from build123d import *

# Parameters (mm, degrees)
BOSS_EXTRUDE3_DEPTH = 3
SKETCH1_5_R         = 8
BOSS_EXTRUDE4_DEPTH = 6
SKETCH1_6_R         = 8
BOSS_EXTRUDE5_DEPTH = 18
SKETCH1_7_R         = 6
CUT_EXTRUDE1_DEPTH  = 12
SKETCH1_8_R         = 3
CUT_EXTRUDE2_DEPTH  = 125


with BuildPart() as part:
    # Sketch1 → Boss-Extrude3 (new body)
    with BuildSketch(Plane(origin=(0, 0, 0), x_dir=(1, 0, 0), z_dir=(0, 1, 0))):
        with BuildLine():
            ThreePointArc((42.894958583, -3.003752345), (37.239092363, 21.5), (18.846153454, 38.65))
            ThreePointArc((18.846153454, 38.65), (16.147655157, 40.973517523), (14.941453584, 44.323995772))
            ThreePointArc((14.941453584, 44.323995772), (0, 58), (-14.941453584, 44.323995772))
            ThreePointArc((-14.941453584, 44.323995772), (-16.147655157, 40.973517523), (-18.846153454, 38.65))
            ThreePointArc((-18.846153454, 38.65), (-37.239092363, 21.5), (-42.894958583, -3.003752345))
            ThreePointArc((-42.894958583, -3.003752345), (-43.557934635, -6.502479184), (-45.856433127, -9.222319513))
            ThreePointArc((-45.856433127, -9.222319513), (-50.229473419, -29), (-30.914979544, -35.101676259))
            ThreePointArc((-30.914979544, -35.101676259), (-27.410279478, -34.471038339), (-24.048805129, -35.646247655))
            ThreePointArc((-24.048805129, -35.646247655), (0, -43), (24.048805129, -35.646247655))
            ThreePointArc((24.048805129, -35.646247655), (27.410279478, -34.471038339), (30.914979544, -35.101676259))
            ThreePointArc((30.914979544, -35.101676259), (50.229473419, -29), (45.856433127, -9.222319513))
            ThreePointArc((45.856433127, -9.222319513), (43.557934635, -6.502479184), (42.894958583, -3.003752345))
        make_face()
        with BuildLine():
            ThreePointArc((-17.531305538, 35.953488372), (-34.641016151, 20), (-39.902287054, -2.794188228))
            ThreePointArc((-39.902287054, -2.794188228), (-40.8493957, -7.792369426), (-44.132964974, -11.67785561))
            ThreePointArc((-44.132964974, -11.67785561), (-47.631397208, -27.5), (-32.179802107, -32.381341007))
            ThreePointArc((-32.179802107, -32.381341007), (-27.173087728, -31.480429693), (-22.370981516, -33.159300144))
            ThreePointArc((-22.370981516, -33.159300144), (0, -40), (22.370981516, -33.159300144))
            ThreePointArc((22.370981516, -33.159300144), (27.173087728, -31.480429693), (32.179802107, -32.381341007))
            ThreePointArc((32.179802107, -32.381341007), (47.631397208, -27.5), (44.132964974, -11.67785561))
            ThreePointArc((44.132964974, -11.67785561), (40.8493957, -7.792369426), (39.902287054, -2.794188228))
            ThreePointArc((39.902287054, -2.794188228), (34.641016151, 20), (17.531305538, 35.953488372))
            ThreePointArc((17.531305538, 35.953488372), (13.676307972, 39.272799119), (11.953162867, 44.059196617))
            ThreePointArc((11.953162867, 44.059196617), (0, 55), (-11.953162867, 44.059196617))
            ThreePointArc((-11.953162867, 44.059196617), (-13.676307972, 39.272799119), (-17.531305538, 35.953488372))
        make_face(mode=Mode.SUBTRACT)
    extrude(amount=BOSS_EXTRUDE3_DEPTH)

    # Sketch1<5> → Boss-Extrude4 (add)
    with BuildSketch(Plane(origin=(0, 0, 0), x_dir=(1, 0, 0), z_dir=(0, 1, 0))):
        with BuildLine():
            ThreePointArc((-17.531305538, 35.953488372), (-13.676307972, 39.272799119), (-11.953162867, 44.059196617))
            ThreePointArc((-11.953162867, 44.059196617), (0, 55), (11.953162867, 44.059196617))
            ThreePointArc((11.953162867, 44.059196617), (13.676307972, 39.272799119), (17.531305538, 35.953488372))
            ThreePointArc((17.531305538, 35.953488372), (34.641016151, 20), (39.902287054, -2.794188228))
            ThreePointArc((39.902287054, -2.794188228), (40.8493957, -7.792369426), (44.132964974, -11.67785561))
            ThreePointArc((44.132964974, -11.67785561), (47.631397208, -27.5), (32.179802107, -32.381341007))
            ThreePointArc((32.179802107, -32.381341007), (27.173087728, -31.480429693), (22.370981516, -33.159300144))
            ThreePointArc((22.370981516, -33.159300144), (0, -40), (-22.370981516, -33.159300144))
            ThreePointArc((-22.370981516, -33.159300144), (-27.173087728, -31.480429693), (-32.179802107, -32.381341007))
            ThreePointArc((-32.179802107, -32.381341007), (-47.631397208, -27.5), (-44.132964974, -11.67785561))
            ThreePointArc((-44.132964974, -11.67785561), (-40.8493957, -7.792369426), (-39.902287054, -2.794188228))
            ThreePointArc((-39.902287054, -2.794188228), (-34.641016151, 20), (-17.531305538, 35.953488372))
        make_face()
        with Locations((37.239092363, -21.5)):
            Circle(SKETCH1_5_R, mode=Mode.SUBTRACT)
        with Locations((-37.239092363, -21.5)):
            Circle(SKETCH1_5_R, mode=Mode.SUBTRACT)
        with Locations((0, 43)):
            Circle(SKETCH1_5_R, mode=Mode.SUBTRACT)
    extrude(amount=BOSS_EXTRUDE4_DEPTH)

    # Sketch1<6> → Boss-Extrude5 (add)
    with BuildSketch(Plane(origin=(0, 0, 0), x_dir=(1, 0, 0), z_dir=(0, 1, 0))):
        with Locations((0, 43)):
            Circle(SKETCH1_6_R)
        with Locations((-37.239092363, -21.5)):
            Circle(SKETCH1_6_R)
        with Locations((37.239092363, -21.5)):
            Circle(SKETCH1_6_R)
    extrude(amount=BOSS_EXTRUDE5_DEPTH)

    # Sketch1<7> → Cut-Extrude1 (cut)
    with BuildSketch(Plane(origin=(0, 0, 0), x_dir=(1, 0, 0), z_dir=(0, 1, 0))):
        with Locations((0, 43)):
            Circle(SKETCH1_7_R)
        with Locations((37.239092363, -21.5)):
            Circle(SKETCH1_7_R)
        with Locations((-37.239092363, -21.5)):
            Circle(SKETCH1_7_R)
    extrude(amount=CUT_EXTRUDE1_DEPTH, mode=Mode.SUBTRACT)

    # Sketch1<8> → Cut-Extrude2 (cut)
    with BuildSketch(Plane(origin=(0, 0, 0), x_dir=(1, 0, 0), z_dir=(0, 1, 0))):
        with Locations((0, 43)):
            Circle(SKETCH1_8_R)
        with Locations((-37.239092363, -21.5)):
            Circle(SKETCH1_8_R)
        with Locations((37.239092363, -21.5)):
            Circle(SKETCH1_8_R)
    extrude(amount=CUT_EXTRUDE2_DEPTH, mode=Mode.SUBTRACT)


solid = part.part
Part model, mm, in its own coordinate system. A direction names the side the tool comes from. Give positions to 0.01 mm unless a question says otherwise; leave off trailing zeros. Loops run counter-clockwise (first coordinate to the right, second up) from the corner with the lowest first, then second, coordinate; pieces in that order, holes last. Notation, with made-up numbers: (-4, 30) -> (42, 30) arc R28 cw to (42, 59) -> close; hole circle Ø5 at (23.25, -32.75). An arc over 180 degrees is marked (long way). Write each question's results on one line, items separated by ' | '. Start each with the question number.
Q1. Which spindle directions (+Z, -Z, +X, -X, +Y, -Y) get a long thin tool onto all of the face, cutting with end or side? Do faces 5 (the face through (0, 4, -55)), 6 (the face through (34, 12, 23)), 7 (the face through (-29.849, 11.916, 24.564)). Say none if no direction does.
Q2. Band-saw the part on B-B on x = 0. List the corners of the cut face in (y, z), plus the area to 3 significant figures.
Q3. Pin check, flat tips, straight feed: P1, Ø7, axis at x = -37.24, z = 21.5, coming from the -Y side; P2, Ø5, axis at x = 6.5, z = 12.5, coming from the +Y side; P3, Ø2, axis at y = 8.5, z = 10.5, coming from the +X side; P4, Ø1.5, axis at y = 9.5, z = 26.5, coming from the -X side. Stop position of each tip, or through.
Q4. Band-saw the part on C-C on z = 21.5. Count the separate pieces of the cut face and the enclosed holes in it, plus the area to 3 significant figures.
Q5. Band-saw the part on A-A on y = 8.5. List the corners of the cut face in (x, z), plus the area to 3 significant figures.
Q6. Wall check: L1, parallel to X at y = 8.5, z = 21.5; L2, parallel to X at y = 16.25, z = 20.5; L3, parallel to X at y = 1.5, z = -38. Give the ranges that are in metal, low to high.
Q7. Band-saw the part on D-D on y = 15.25. List the corners of the cut face in (x, z).
Q8. Pull direction X, two halves, no side cores. Call faces 1 (the face through (43.58, 1.48, 6.55)), 2 (the face through (42.962, 5.916, 19.698)), 3 (the face through (-37.89, 14.96, 24.43)), 4 (the face through (-34.806, 4.479, -19.711)): +X half, -X half, draft (parallel to the pull), parting line (faces both ways), or undercut.
Results are:
1) face 5: -Z, +Y | face 6: -Y | face 7: +Y
2) outline: (0, -58) -> (3, -58) -> (3, -55) -> (6, -55) -> (6, -51) -> (18, -51) -> (18, -46) -> (12, -46) -> (12, -49) -> (0, -49) -> close; (0, -37) -> (12, -37) -> (12, -40) -> (18, -40) -> (18, -35) -> (6, -35) -> (6, 40) -> (3, 40) -> (3, 43) -> (0, 43) -> close | area: 600 mm²
3) P1: stops at y = 12 | P2: stops at y = 6 | P3: passes through | P4: stops at x = -44.02
4) separate pieces: 3 | enclosed holes: 0 | area: 633 mm²
5) outline: circle Ø16 at (-37.24, 21.5); circle Ø16 at (0, -43); circle Ø16 at (37.24, 21.5); hole circle Ø12 at (-37.24, 21.5); hole circle Ø12 at (0, -43); hole circle Ø12 at (37.24, 21.5) | area: 264 mm²
6) L1: x = -45.24 to -43.24, -31.24 to -29.24, 29.24 to 31.24, 43.24 to 45.24 | L2: x = -45.18 to -40.07, -34.41 to -29.3, 29.3 to 34.41, 40.07 to 45.18 | L3: x = -20.12 to -3.32, 3.32 to 20.12
7) outline: circle Ø16 at (-37.24, 21.5); circle Ø16 at (0, -43); circle Ø16 at (37.24, 21.5); hole circle Ø6 at (-37.24, 21.5); hole circle Ø6 at (0, -43); hole circle Ø6 at (37.24, 21.5)
8) face 1: +X half | face 2: undercut | face 3: undercut | face 4: -X half
